from build123d import *

# Parameters (mm, degrees)
BOSS_EXTRUDE1_DEPTH = 25
SKETCH2_R           = 11.05
CUT_EXTRUDE1_DEPTH  = 7
CUT_EXTRUDE3_DEPTH  = 8.75
CUT_EXTRUDE5_DEPTH  = 8.75
SKETCH5_R           = 1
CUT_EXTRUDE6_DEPTH  = 7.5
SKETCH6_R           = 1.95
CUT_EXTRUDE7_DEPTH  = 6.5
SKETCH7_R           = 2
CUT_EXTRUDE8_DEPTH  = 1
CUT_EXTRUDE9_DEPTH  = 62.065538563
CUT_EXTRUDE10_DEPTH = 3.5


with BuildPart() as part:
    # Sketch1 → Boss-Extrude1 (new body)
    with BuildSketch(Plane(origin=(0, 0, 0), x_dir=(1, 0, 0), z_dir=(0, 1, 0))):
        with BuildLine():
            Line((-42, -10), (42, -10))
            ThreePointArc((42, -10), (52, 0), (42, 10))
            Line((42, 10), (-42, 10))
            ThreePointArc((-42, 10), (-52, 0), (-42, -10))
        make_face()
    extrude(amount=BOSS_EXTRUDE1_DEPTH)

    # Sketch2 → Cut-Extrude1 (cut)
    with BuildSketch(Plane.XY.offset(10)):
        with Locations((0, 12.5)):
            Circle(SKETCH2_R)
    extrude(amount=-CUT_EXTRUDE1_DEPTH, mode=Mode.SUBTRACT)

    # Sketch3 → Cut-Extrude3 (cut)
    with BuildSketch(Plane.XZ):
        with BuildLine():
            Line((15, -10), (15, 10))
            Line((15, 10), (42, 10))
            ThreePointArc((42, 10), (52, 0), (42, -10))
            Line((42, -10), (15, -10))
        make_face()
        with BuildLine():
            Line((-15, -10), (-15, 10))
            Line((-15, 10), (-42, 10))
            ThreePointArc((-42, 10), (-52, 0), (-42, -10))
            Line((-42, -10), (-15, -10))
        make_face()
    extrude(amount=-CUT_EXTRUDE3_DEPTH, mode=Mode.SUBTRACT)

    # Sketch4 → Cut-Extrude5 (cut)
    with BuildSketch(Plane(origin=(0, 25, 0), x_dir=(1, 0, 0), z_dir=(0, 1, 0))):
        with BuildLine():
            Line((15, -10), (15, 10))
            Line((15, 10), (55, 10))
            ThreePointArc((55, 10), (65, 0), (55, -10))
            Line((55, -10), (15, -10))
        make_face()
        with BuildLine():
            Line((-15, -10), (-15, 10))
            Line((-15, 10), (-55, 10))
            ThreePointArc((-55, 10), (-65, 0), (-55, -10))
            Line((-55, -10), (-15, -10))
        make_face()
    extrude(amount=-CUT_EXTRUDE5_DEPTH, mode=Mode.SUBTRACT)

    # Sketch5 → Cut-Extrude6 (cut)
    with BuildSketch(Plane(origin=(0, 16.25, 0), x_dir=(1, 0, 0), z_dir=(0, 1, 0))):
        with Locations(Location((-42, 6.2, 0), (0, 0, 270))):
            Circle(SKETCH5_R)
        with Locations(Location((-35.8, 0, 0), (0, 0, 270))):
            Circle(SKETCH5_R)
        with Locations(Location((-42, -6.2, 0), (0, 0, 270))):
            Circle(SKETCH5_R)
        with Locations(Location((-48.2, 0, 0), (0, 0, 270))):
            Circle(SKETCH5_R)
        with Locations(Location((42, 6.2, 0), (0, 0, 270))):
            Circle(SKETCH5_R)
        with Locations(Location((48.2, 0, 0), (0, 0, 270))):
            Circle(SKETCH5_R)
        with Locations(Location((42, -6.2, 0), (0, 0, 270))):
            Circle(SKETCH5_R)
        with Locations(Location((35.8, 0, 0), (0, 0, 270))):
            Circle(SKETCH5_R)
    extrude(amount=-CUT_EXTRUDE6_DEPTH, mode=Mode.SUBTRACT)

    # Sketch6 → Cut-Extrude7 (cut)
    with BuildSketch(Plane.XZ.offset(-8.75)):
        with Locations(Location((-42, 6.2, 0), (0, 0, 270))):
            Circle(SKETCH6_R)
        with Locations(Location((-35.8, 0, 0), (0, 0, 270))):
            Circle(SKETCH6_R)
        with Locations(Location((-48.2, 0, 0), (0, 0, 270))):
            Circle(SKETCH6_R)
        with Locations(Location((-42, -6.2, 0), (0, 0, 270))):
            Circle(SKETCH6_R)
        with Locations(Location((42, 6.2, 0), (0, 0, 270))):
            Circle(SKETCH6_R)
        with Locations(Location((48.2, 0, 0), (0, 0, 270))):
            Circle(SKETCH6_R)
        with Locations(Location((35.8, 0, 0), (0, 0, 270))):
            Circle(SKETCH6_R)
        with Locations(Location((42, -6.2, 0), (0, 0, 270))):
            Circle(SKETCH6_R)
    extrude(amount=-CUT_EXTRUDE7_DEPTH, mode=Mode.SUBTRACT)

    # Sketch7 → Cut-Extrude8 (cut)
    with BuildSketch(Plane(origin=(0, 16.25, 0), x_dir=(1, 0, 0), z_dir=(0, 1, 0))):
        with Locations(Location((-42, 0, 0), (0, 0, 270))):
            Circle(SKETCH7_R)
        with Locations(Location((42, 0, 0), (0, 0, 270))):
            Circle(SKETCH7_R)
    extrude(amount=-CUT_EXTRUDE8_DEPTH, mode=Mode.SUBTRACT)

    # Sketch8 → Cut-Extrude9 (cut, through all)
    with BuildSketch(Plane.XY.offset(10)):
        with BuildLine():
            Line((-15, 16.25), (-15, 25))
            Line((-15, 25), (-9.100137362, 25))
            ThreePointArc((-9.100137362, 25), (-12.819702813, 21.143941218), (-15, 16.25))
        make_face()
        with BuildLine():
            Line((15, 0), (9.100137362, 0))
            ThreePointArc((9.100137362, 0), (12.819702813, 3.856058782), (15, 8.75))
            Line((15, 8.75), (15, 0))
        make_face()
        with BuildLine():
            Line((15, 25), (9.100137362, 25))
            ThreePointArc((9.100137362, 25), (12.819702813, 21.143941218), (15, 16.25))
            Line((15, 16.25), (15, 25))
        make_face()
        with BuildLine():
            Line((-15, 0), (-15, 8.75))
            ThreePointArc((-15, 8.75), (-12.819702813, 3.856058782), (-9.100137362, 0))
            Line((-9.100137362, 0), (-15, 0))
        make_face()
    extrude(amount=-CUT_EXTRUDE9_DEPTH, mode=Mode.SUBTRACT)

    # Sketch9 → Cut-Extrude10 (cut)
    with BuildSketch(Plane.XY.offset(3)):
        with BuildLine():
            Line((0.5, 10), (0.5, 7.525062814))
            ThreePointArc((0.5, 7.525062814), (5, 12.5), (0.5, 17.474937186))
            Line((0.5, 17.474937186), (0.5, 15))
            Line((0.5, 15), (-0.5, 15))
            Line((-0.5, 15), (-0.5, 17.474937186))
            ThreePointArc((-0.5, 17.474937186), (-5, 12.5), (-0.5, 7.525062814))
            Line((-0.5, 7.525062814), (-0.5, 10))
            Line((-0.5, 10), (0.5, 10))
        make_face()
    extrude(amount=-CUT_EXTRUDE10_DEPTH, mode=Mode.SUBTRACT)


solid = part.part
Work out the finished part from the listing and answer in its coordinate system (mm). A direction names the side the tool comes from. Give positions to 0.01 mm unless a question says otherwise; leave off trailing zeros. Loops run counter-clockwise (first coordinate to the right, second up) from the corner with the lowest first, then second, coordinate; pieces in that order, holes last. Notation, with made-up numbers: (71, -39) -> (91, -39) arc R20 cw to (91, -31) -> close; hole circle Ø4 at (23.5, 71.25). An arc over 180 degrees is marked (long way). Use a Markdown table: item, result. Add a question column.
1. Section C-C on z = -6.2 is taken. Determine the outline of the cut face in (x, y), and give its area (3 significant figures).
2. Find the intervals of material crossed by probe 1 along X at (y, z) = (11, 0); probe 2 along Z at (x, y) = (0.5, 10.75); probe 3 along Y at (x, z) = (-22, 6.5), in increasing order.
3. For faces 4 (the flat face through (34, 8.75, -2)), 5 (the flat face through (-34, 16.25, 0)), 6 (the cylindrical face through (-50.104, 11.954, 0.423)), 7 (the flat face through (34, 16.25, 0)), determine the directions among +Z, -Z, +X, -X, +Y, -Y from which every point of the face is accessible in a straight line to the end or side of a thin tool.
4. Flat-ended cylindrical pins translate along their axes: pin 1 Ø4.5 at (x, z) = (42, 0) entering from +Y; pin 2 Ø0.7 at (y, z) = (9.5, 1.5) entering from -X; pin 3 Ø1 at (x, z) = (-31.5, -2) entering from -Y; pin 4 Ø12 at (x, y) = (21.5, 19) entering from -Z. Find the tip coordinate at first contact, or state that the pin passes through.
5. Section D-D on x = 3.5 is taken. Determine the outline of the cut face in (y, z).
6. Section A-A on x = -35.8 is taken. Determine the outline of the cut face in (y, z).
7. Section B-B on y = 4.25 is taken. Determine the outline of the cut face in (x, z).
8. Determine the mould class of faces 1 (the cylindrical face through (12.777, 3.794, 0.14)), 2 (the cylindrical face through (-41.01, 15.76, -6.33)), 3 (the flat face through (0, 25, 0)) for opening direction X: released by +X, released by -X, zero draft, split by the parting line, or undercut.
Results below:
| question | item | result |
|---|---|---|
| 1 | outline | (-49.85, 8.75) -> (-43.95, 8.75) -> (-43.95, 15.25) -> (-43, 15.25) -> (-43, 16.25) -> (-49.85, 16.25) -> close; (-41, 15.25) -> (-40.05, 15.25) -> (-40.05, 8.75) -> (-15, 8.75) arc R15.46 ccw to (-9.1, 0) -> (9.1, 0) arc R15.46 ccw to (15, 8.75) -> (40.05, 8.75) -> (40.05, 15.25) -> (41, 15.25) -> (41, 16.25) -> (15, 16.25) arc R15.46 ccw to (9.1, 25) -> (-9.1, 25) arc R15.46 ccw to (-15, 16.25) -> (-41, 16.25) -> close; (43, 15.25) -> (43.95, 15.25) -> (43.95, 8.75) -> (49.85, 8.75) -> (49.85, 16.25) -> (43, 16.25) -> close |
| 1 | area | 1,140 mm^2 |
| 2 | probe 1 | x = -52 to -50.15, -46.25 to -37.75, -33.85 to -4.77, 4.77 to 33.85, 37.75 to 46.25, 50.15 to 52 |
| 2 | probe 2 | z = -10 to -0.5 |
| 2 | probe 3 | y = 8.75 to 16.25 |
| 3 | face 4 | +Z, -Z, +X, -Y |
| 3 | face 5 | +Z, -Z, -X, +Y |
| 3 | face 6 | -Y |
| 3 | face 7 | +Z, -Z, +X, +Y |
| 4 | pin 1 | stops at y = 16.25 |
| 4 | pin 2 | stops at x = -51.93 |
| 4 | pin 3 | stops at y = 8.75 |
| 4 | pin 4 | stops at z = -10 |
| 5 | outline | (0, -10) -> (25, -10) -> (25, 10) -> (22.98, 10) -> (22.98, 3) -> (16.07, 3) -> (16.07, -0.5) -> (8.93, -0.5) -> (8.93, 3) -> (2.02, 3) -> (2.02, 10) -> (0, 10) -> close |
| 6 | outline | (8.75, -10) -> (16.25, -10) -> (16.25, -1) -> (15.25, -1) -> (15.25, -1.95) -> (8.75, -1.95) -> close; (8.75, 1.95) -> (15.25, 1.95) -> (15.25, 1) -> (16.25, 1) -> (16.25, 10) -> (8.75, 10) -> close |
| 7 | outline | (-13.08, -10) -> (13.08, -10) -> (13.08, 10) -> (7.35, 10) -> (7.35, 3) -> (-7.35, 3) -> (-7.35, 10) -> (-13.08, 10) -> close |
| 8 | face 1 | released by +X |
| 8 | face 2 | undercut |
| 8 | face 3 | zero draft |
